Check sheet for the drawn part. Datum: minimum x, y, z corner. Units: mm. A direction names the side the tool comes from. Coordinates: 2 decimals unless noted, no trailing zeros. Order: outer loops, then holes, each group sorted by start corner. A loop starts at its lowest first (then second) coordinate and runs counter-clockwise, first axis right, second up.
1. Cross-section at D-D (x = 25). Enter the section's corners in (y, z).
2. Set-up check for the marked faces 5, 6 and 7: record each of +Z, -Z, +X, -X, +Y, -Y from which the full face is reachable in a straight line by a thin tool's end or side.
3. Draft check along X on the marked faces 1, 2, 3 and 4. Enter one of: released by +X, released by -X, zero draft, split by the parting line, or undercut.
4. Thickness scan on line 1 (X direction, y = 4.5, z = 6) (1 decimal); line 2 (X direction, y = 30.5, z = 2) (1 decimal); line 3 (Y direction, x = 11, z = 6.75). Record the ranges inside material, lowest first.
5. Cross-section at B-B (y = 6.5). Enter the section's corners in (x, z) (1 decimal), then the cut area to 3 significant figures.
6. Cross-section at A-A (z = 1.5). Enter the section's corners in (x, y) (1 decimal).
7. Cross-section at C-C (y = 39.3). Enter the section's corners in (x, z), then the cut area to 3 significant figures.
8. Gauge pin test, flat ends, axial feed: pin 1 Ø2 at (x, y) = (50.02, 31.5) entering from +Z; pin 2 Ø2.5 at (y, z) = (46.5, 2.5) entering from +X; pin 3 Ø2.5 at (x, y) = (51.02, 39.3) entering from -Z; pin 4 Ø3.5 at (x, y) = (30.5, 11) entering from -Z. Record the tip position at first contact, or that the pin passes through.
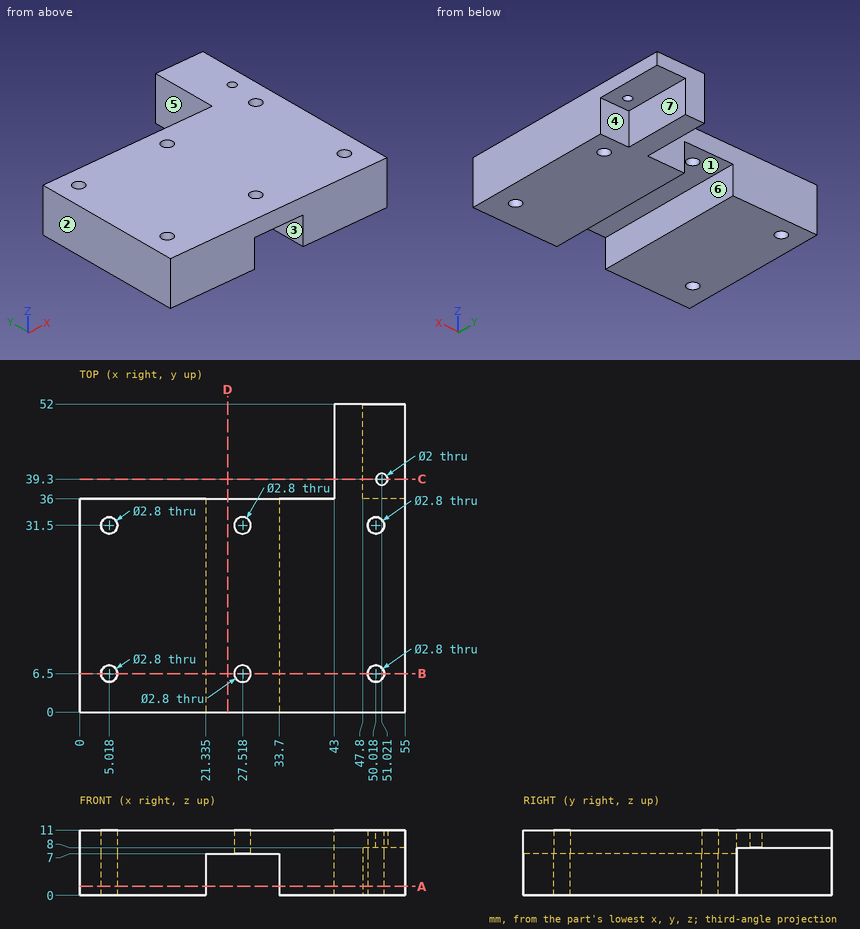
Data:
1. outline: (0, 7) - (36, 7) - (36, 11) - (0, 11) - close
2. face 5: +Z, -Z, -X, +Y
2. face 6: -Z, +Y, -Y
2. face 7: -Z, +X, +Y
3. face 1: undercut
3. face 2: released by -X
3. face 3: undercut
3. face 4: zero draft
4. line 1: x = 0 to 21.3, 33.7 to 55
4. line 2: x = 0 to 4, 6 to 21.3, 33.7 to 49, 51 to 55
4. line 3: y = 0 to 36
5. outline: (0, 0) - (3.6, 0) - (3.6, 11) - (0, 11) - close; (6.4, 0) - (21.3, 0) - (21.3, 7) - (26.1, 7) - (26.1, 11) - (6.4, 11) - close; (28.9, 7) - (33.7, 7) - (33.7, 0) - (48.6, 0) - (48.6, 11) - (28.9, 11) - close; (51.4, 0) - (55, 0) - (55, 11) - (51.4, 11) - close
5. area: 446 mm2
6. outline: (0, 0) - (21.3, 0) - (21.3, 36) - (0, 36) - close; (33.7, 0) - (55, 0) - (55, 36) - (47.8, 36) - (47.8, 52) - (43, 52) - (43, 36) - (33.7, 36) - close; hole circle Ø2.8 at (5, 6.5); hole circle Ø2.8 at (5, 31.5); hole circle Ø2.8 at (50, 6.5); hole circle Ø2.8 at (50, 31.5)
7. outline: (43, 0) - (47.8, 0) - (47.8, 8) - (50.02, 8) - (50.02, 11) - (43, 11) - close; (52.02, 8) - (55, 8) - (55, 11) - (52.02, 11) - close
7. area: 68.4 mm2
8. pin 1: passes through
8. pin 2: stops at x = 47.8
8. pin 3: stops at z = 8
8. pin 4: stops at z = 7
